Build history of the part. All positions in model axes, mm. A direction names the side the tool comes from. Give positions to 0.01 mm unless a question says otherwise; leave off trailing zeros. Write each loop counter-clockwise with the first axis right and the second up, starting at its lowest first coordinate (ties: lowest second). Pieces come first, ordered by that corner, then holes.
Autodesk Inventor part; units mm, degrees
ref_plane "YZ Plane" through (0, 0, 0) normal (1, 0, 0) x (0, 1, 0)
ref_plane "XZ Plane" through (0, 0, 0) normal (0, 1, 0) x (-1, 0, 0)
ref_plane "XY Plane" through (0, 0, 0) normal (0, 0, 1) x (1, 0, 0)
sketch "Skizze4" plane through (0, 0, 0) normal (0, 0, 1) x (1, 0, 0)
  line L0 (15, 15) -> (-15, 15)
  line L1 (-15, 15) -> (-15, 0)
  line L2 (-15, -15) -> (15, 15) construction
  line L3 (15, -15) -> (-15, 15) construction
  line L4 (-15, 0) -> (15, 0)
  arc A0 (13, 0) -> (-13, 0) centre (0, 0) ccw
  line L5 (15, 0) -> (15, 15)
  dimension "d9" = 30
  dimension "d10" = 30
extrude "Extrusion4" add sketch "Skizze4" along normal blind 30 contours L5 L4 A0 L1 L0
sketch "Skizze5" plane through (0, 0, 0) normal (0, 0, -1) x (-1, 0, 0)
  line L0 (-15, 0) -> (-15, 15)
  line L1 (15, 0) -> (13, 0)
  line L2 (-15, 15) -> (15, 15)
  line L3 (15, 15) -> (15, 0)
  line L4 (15, 0) -> (-15, 0)
  line L5 (-15, 0) -> (-15, 15)
  point P0 (0, 0)
extrude "Extrusion5" add sketch "Skizze5" along normal blind 2
sketch "Skizze6" plane through (0, 0, -2) normal (0, 0, -1) x (-1, 0, 0)
  line L0 (-15, 0) -> (-15, 15)
  line L1 (15, 0) -> (13, 0)
  line L2 (-15, 15) -> (15, 15)
  line L3 (15, 15) -> (15, 0)
  line L4 (15, 0) -> (-15, 0)
  line L5 (-15, 0) -> (-15, 15)
  arc A0 (13, 0) -> (-13, 0) centre (0, 0) ccw
  dimension "d16" = 26
extrude "Extrusion6" add sketch "Skizze6" along normal blind 30 contours L0 L2 L3 L1 A0 L4
sketch "Skizze9" plane through (15, 0, 30) normal (1, 0, 0) x (0, 0, -1)
  line L0 (0, 0) -> (0, 13)
  line L1 (62, 13) -> (62, 0)
  line L2 (62, 0) -> (0, 0)
  line L3 (23.5, 2) -> (38.5, 2)
  line L4 (38.5, 2) -> (38.5, 0)
  line L5 (38.5, 0) -> (23.5, 0)
  line L6 (23.5, 0) -> (23.5, 2)
  line L7 (23.5, 2) -> (38.5, 0) construction
  line L8 (38.5, 2) -> (23.5, 0) construction
  point P0 (30, 0)
  point P1 (31, 1)
  dimension "d36" = 15
extrude "Extrusion8" add sketch "Skizze9" along normal blind 15
sketch "Skizze10" plane through (-15, 0, 30) normal (-1, 0, 0) x (0, 0, 1)
  line L0 (0, 0) -> (0, 15)
  line L1 (0, 6.5004) -> (31, 6.5004) construction
  line L2 (0, 0) -> (-62, 0)
  line L3 (-31, 0) -> (-31, 1)
  line L4 (-38.5, 2) -> (-23.5, 2)
  line L5 (-23.5, 2) -> (-23.5, 0)
  line L6 (-23.5, 0) -> (-38.5, 0)
  line L7 (-38.5, 0) -> (-38.5, 2)
  line L8 (-38.5, 2) -> (-23.5, 0) construction
  line L9 (-23.5, 2) -> (-38.5, 0) construction
  point P0 (-30, 0)
  dimension "d41" = 1
  dimension "d42" = 15
  dimension "d43" = 2
extrude "Extrusion9" add sketch "Skizze10" along normal blind 15
sketch "Skizze11" plane through (-15, 15, 30) normal (0, 1, 0) x (1, 0, 0)
  line L0 (0, 23.5) -> (-15, 23.5)
  line L1 (0, 62) -> (0, 0)
  line L2 (30, 62) -> (30, 0)
  line L3 (23, 22) -> (7, 22)
  line L4 (7, 22) -> (7, 18)
  line L5 (7, 18) -> (23, 18)
  line L6 (23, 18) -> (23, 22)
  line L7 (23, 22) -> (7, 18) construction
  line L8 (7, 22) -> (23, 18) construction
  line L9 (7, 44) -> (23, 44)
  line L10 (23, 44) -> (23, 40)
  line L11 (23, 40) -> (7, 40)
  line L12 (7, 40) -> (7, 44)
  line L13 (7, 44) -> (23, 40) construction
  line L14 (23, 44) -> (7, 40) construction
  point P0 (15, 30)
  dimension "d55" = 16
  dimension "d56" = 4
  dimension "d58" = 16
  dimension "d59" = 4
extrude "Extrusion10" cut sketch "Skizze11" against normal through all
sketch "Skizze12" plane through (-15, 2, 6.5) normal (0, 1, 0) x (1, 0, 0)
  line L0 (-15, 15) -> (-15, 0)
  line L1 (0, 38.5) -> (0, -23.5)
  line L2 (-15, 0) -> (6.2132, 0) construction
  circle A0 centre (-7.5, 7.5) radius 2.5
  point P0 (15, 6.5)
  dimension "d63" = 5
extrude "Extrusion11" cut sketch "Skizze12" against normal through all
sketch "Skizze13" plane through (15, 2, 6.5) normal (0, 1, 0) x (1, 0, 0)
  line L0 (0, 0) -> (15, 0)
  line L1 (0, 38.5) -> (0, -23.5)
  line L2 (15, 0) -> (36.2132, 0) construction
  circle A0 centre (7.5, 7.5) radius 2.5
  point P0 (-15, 6.5)
  dimension "d67" = 5
extrude "Extrusion12" cut sketch "Skizze13" against normal blind 10
sketch "Skizze15" plane through (0, 0, -2) normal (0, 0, -1) x (-1, 0, 0)
  circle A0 centre (0, 0) radius 13
extrude "Extrusion14" cut sketch "Skizze15" against normal blind 2
properties part number "Motorhalterung_Teil2"
1. Mould opens along X. For faces 6 (the face through (-4, 13, 30)), 7 (the face through (0, 13, -1)), 8 (the face through (30, 1, -1)) say: pulls with the +X half, pulls with the -X half, needs draft (parallel to the pull), parting line crosses it, or undercut.
2. Drill centre lines: line 1 along X through (y, z) = (0.65, -1); line 2 along Z through (x, y) = (-22.5, 0.75); line 3 along X through (y, z) = (10.25, 19). Where is each one in solid material? Low to high.
3. Saw through at A-A on y = 12. Give the cut face in (x, z).
4. Saw through at B-B on y = 1.25. Give the cut face in (x, z), plus the area to 3 significant figures.
5. Drop flat-ended pins along their axis: pin 1 (3 mm diameter, centred on y = 13.5, z = 10.5, fed in from -X); pin 2 (3 mm diameter, centred on y = 13, z = -12.5, fed in from +X); pin 3 (1 mm diameter, centred on x = -22, y = 1, fed in from -Z); pin 4 (8 mm diameter, centred on x = -6.5, y = 6, fed in from -Z). Give the stop position or say it passes through.
6. 3-axis set-ups, long thin cutter, end or side, ignore diameter. For faces 1 (the face through (-22, 1, -8.5)), 2 (the face through (19, 2, -1)), 3 (the face through (0, 14, -14)), 4 (the face through (22, 1, -8.5)), 5 (the face through (22, 1, 6.5)): which of +Z, -Z, +X, -X, +Y, -Y reach the whole face in a straight line?
7. Saw through at C-C on x = 22.5. Give the cut face in (y, z), plus the area to 3 significant figures.
8. Saw through at D-D on z = -1. Give the cut face in (x, y).
Outcome:
1. face 6: needs draft
1. face 7: undercut
1. face 8: pulls with the +X half
2. line 1: x = -30 to -25, -20 to -12.98, 12.98 to 20, 25 to 30
2. line 2: z = -8.5 to -3.5, 1.5 to 6.5
2. line 3: x = -15 to -8, 8 to 15
3. outline: (-15, -32) - (-5, -32) - (-5, -14) - (-8, -14) - (-8, -10) - (-5, -10) - (-5, 8) - (-8, 8) - (-8, 12) - (-5, 12) - (-5, 30) - (-15, 30) - close; (5, -32) - (15, -32) - (15, 30) - (5, 30) - (5, 12) - (8, 12) - (8, 8) - (5, 8) - (5, -10) - (8, -10) - (8, -14) - (5, -14) - close
4. outline: (-30, -8.5) - (-15, -8.5) - (-15, -32) - (-12.94, -32) - (-12.94, 30) - (-15, 30) - (-15, 6.5) - (-30, 6.5) - close; (12.94, -32) - (15, -32) - (15, -8.5) - (30, -8.5) - (30, 6.5) - (15, 6.5) - (15, 30) - (12.94, 30) - close; hole circle Ø5 at (-22.5, -1); hole circle Ø5 at (22.5, -1)
4. area: 666 mm2
5. pin 1: stops at x = -15
5. pin 2: stops at x = 15
5. pin 3: stops at z = -8.5
5. pin 4: passes through
6. face 1: -Z, -X, +Y, -Y
6. face 2: +Z, -Z, +X, +Y
6. face 3: +Y, -Y
6. face 4: -Z, +X, +Y, -Y
6. face 5: +Z, +X, +Y, -Y
7. outline: (0, -8.5) - (2, -8.5) - (2, -3.5) - (0, -3.5) - close; (0, 1.5) - (2, 1.5) - (2, 6.5) - (0, 6.5) - close
7. area: 20.0 mm2
8. outline: (-30, 0) - (-25, 0) - (-25, 2) - (-30, 2) - close; (-20, 0) - (-13, 0) arc R13 cw to (13, 0) - (20, 0) - (20, 2) - (15, 2) - (15, 15) - (-15, 15) - (-15, 2) - (-20, 2) - close; (25, 0) - (30, 0) - (30, 2) - (25, 2) - close
